from build123d import *

# Parameters (mm, degrees)
SKETCH1_W                = 340
SKETCH1_H                = 400
BOSS_EXTRUDE1_DEPTH      = 20
SKETCH2_W                = 20
SKETCH2_H                = 400
BOSS_EXTRUDE2_DEPTH      = 630
SKETCH3_W                = 300
SKETCH3_H                = 400
BOSS_EXTRUDE3_DEPTH      = 10
BOSS_EXTRUDE4_DEPTH      = 20
BOSS_EXTRUDE4_DEPTH_BACK = 420
SKETCH8_W                = 20
SKETCH8_H                = 780
CUT_EXTRUDE4_DEPTH       = 20
FILLET1_R                = 5
SKETCH10_R               = 3
CUT_EXTRUDE5_DEPTH       = 13
SKETCH11_R               = 3
CUT_EXTRUDE6_DEPTH       = 13
MIRROR5_COPY_1_SKETCH_R  = 3
MIRROR5_COPY_1_DEPTH     = 13


with BuildPart() as part:
    # Sketch1 → Boss-Extrude1 (new body)
    with BuildSketch(Plane(origin=(0, 0, 0), x_dir=(1, 0, 0), z_dir=(0, 1, 0))):
        Rectangle(SKETCH1_W, SKETCH1_H)
    boss_extrude1 = extrude(amount=BOSS_EXTRUDE1_DEPTH)

    # Sketch2 → Boss-Extrude2 (add)
    with BuildSketch(Plane(origin=(0, 20, 0), x_dir=(1, 0, 0), z_dir=(0, 1, 0))):
        with Locations((-160, 0)):
            Rectangle(SKETCH2_W, SKETCH2_H)
    boss_extrude2 = extrude(amount=BOSS_EXTRUDE2_DEPTH)

    # Sketch3 → Boss-Extrude3 (add, symmetric)
    with BuildSketch(Plane(origin=(0, 335, 0), x_dir=(1, 0, 0), z_dir=(0, 1, 0))):
        Rectangle(SKETCH3_W, SKETCH3_H)
    extrude(amount=BOSS_EXTRUDE3_DEPTH, both=True)

    # Mirror1: Boss-Extrude1 across plane
    add(boss_extrude1.mirror(Plane.ZX.offset(335)))

    # Mirror2: Boss-Extrude2 across plane
    add(boss_extrude2.mirror(Plane(origin=(0, 0, 0), x_dir=(0, 0, 1), z_dir=(1, 0, 0))))

    # Sketch8 → Boss-Extrude4 (add, two sides: drawn at the far end of the back side and taken through both)
    with BuildSketch(Plane.XY.offset(200).offset(-BOSS_EXTRUDE4_DEPTH_BACK)):
        with Locations((180, 330)):
            Rectangle(SKETCH8_W, SKETCH8_H)
    extrude(amount=BOSS_EXTRUDE4_DEPTH + BOSS_EXTRUDE4_DEPTH_BACK)

    # Sketch9 → Cut-Extrude4 (cut)
    with BuildSketch(Plane(origin=(190, 0, 0), x_dir=(0, 0, -1), z_dir=(1, 0, 0))):
        with BuildLine():
            Line((-60, 720), (-51.823392624, 695.470177872))
            ThreePointArc((-51.823392624, 695.470177872), (-48.911608517, 691.510062519), (-44.23392624, 690))
            Line((-44.23392624, 690), (44.23392624, 690))
            ThreePointArc((44.23392624, 690), (48.911608517, 691.510062519), (51.823392624, 695.470177872))
            Line((51.823392624, 695.470177872), (60, 720))
            Line((60, 720), (-60, 720))
        make_face()
    extrude(amount=-CUT_EXTRUDE4_DEPTH, mode=Mode.SUBTRACT)

    # Fillet1
    fillet1_edges = [part.edges().sort_by_distance(p)[0] for p in [
        (180, 720, 60),
        (180, 720, -60),
    ]]
    fillet(fillet1_edges, radius=FILLET1_R)

    # Sketch10 → Cut-Extrude5 (cut)
    with BuildSketch(Plane.ZY.offset(170)):
        with Locations((174, 628.5)):
            Circle(SKETCH10_R)
        with Locations((142.5, 628.5)):
            Circle(SKETCH10_R)
        with Locations((111, 628.5)):
            Circle(SKETCH10_R)
    cut_extrude5 = extrude(amount=-CUT_EXTRUDE5_DEPTH, mode=Mode.SUBTRACT)

    # Mirror3: Cut-Extrude5 across plane
    add(cut_extrude5.mirror(Plane.XY), mode=Mode.SUBTRACT)

    # Sketch11 → Cut-Extrude6 (cut)
    with BuildSketch(Plane.XZ):
        with Locations(Location((-124, -140, 0), (0, 0, 270))):
            Circle(SKETCH11_R)
        with Locations(Location((-76, -140, 0), (0, 0, 270))):
            Circle(SKETCH11_R)
    cut_extrude6 = extrude(amount=-CUT_EXTRUDE6_DEPTH, mode=Mode.SUBTRACT)

    # Mirror4: Cut-Extrude6 across plane
    add(cut_extrude6.mirror(Plane(origin=(0, 0, 0), x_dir=(0, 0, 1), z_dir=(1, 0, 0))), mode=Mode.SUBTRACT)

    # Mirror5: Cut-Extrude6 across plane
    add(cut_extrude6.mirror(Plane.XY), mode=Mode.SUBTRACT)

    # Mirror5 copy 1 sketch → Mirror5 copy 1 (cut)
    with BuildSketch(Plane(origin=(0, 0, 0), x_dir=(-1, 0, 0), z_dir=(0, -1, 0))):
        with Locations(Location((-124, -140, 0), (0, 0, 270))):
            Circle(MIRROR5_COPY_1_SKETCH_R)
        with Locations(Location((-76, -140, 0), (0, 0, 270))):
            Circle(MIRROR5_COPY_1_SKETCH_R)
    extrude(amount=-MIRROR5_COPY_1_DEPTH, mode=Mode.SUBTRACT)


solid = part.part
Part model, mm, in its own coordinate system. A direction names the side the tool comes from. Give positions to 0.01 mm unless a question says otherwise; leave off trailing zeros. Order: outer loops, then holes, each group sorted by start corner. A loop starts at its lowest first (then second) coordinate and runs counter-clockwise, first axis right, second up. Notation, with made-up numbers: (51, 80) - (66, 80) arc R19 cw to (66, 110) - close; hole circle Ø1 at (-29.75, 84). An arc over 180 degrees is marked (long way). Use a Markdown table: item, result.
1) Saw through at B-B on x = -41. List the corners of the cut face in (y, z), plus the area to 3 significant figures.
Checked values:
| item | result |
|---|---|
| outline | (0, -200) - (20, -200) - (20, 200) - (0, 200) - close; (325, -200) - (345, -200) - (345, 200) - (325, 200) - close; (650, -200) - (670, -200) - (670, 200) - (650, 200) - close |
| area | 24,000 mm² |
2) Flat gauge pins, fed straight in: P1, Ø7, axis at x = 124, z = -140, coming from the +Y side; P2, Ø1.8, axis at y = 629.5, z = -173.5, coming from the -X side; P3, Ø4, axis at x = -105.5, z = -87.5, coming from the -Y side. Where does each tip first touch, or does it go through?
Checked values:
| item | result |
|---|---|
| P1 | y = 670 |
| P2 | x = -157 |
| P3 | y = 0 |
3) Two-plate mould, pull along Y, no slides. Class faces 1 (the flat face through (180.1, 705.9, -55.3)), 2 (the flat face through (150, 170, 3)), 3 (the flat face through (190, 325, -3)): +Y half, -Y half, draft (parallel to the pull), parting line (faces both ways), or undercut.
Checked values:
| item | result |
|---|---|
| face 1 | +Y half |
| face 2 | undercut |
| face 3 | draft |
4) 3-axis set-ups, long thin cutter, end or side, ignore diameter. For faces 4 (the flat face through (170, 270, 211)), 5 (the flat face through (1, 333, 200)), 6 (the flat face through (1, 333, -200)), 7 (the flat face through (180.1, 706.2, 55.4)), 8 (the flat face through (-150, 495, 3)): which of +Z, -Z, +X, -X, +Y, -Y reach the whole face in a straight line?
Checked values:
| item | result |
|---|---|
| face 4 | -X |
| face 5 | +Z, -X, +Y, -Y |
| face 6 | -Z, -X, +Y, -Y |
| face 7 | +X, -X, +Y |
| face 8 | +Z, -Z |
5) Saw through at C-C on z = -157.5. List the corners of the cut face in (x, y), plus the area to 3 significant figures.
Checked values:
| item | result |
|---|---|
| outline | (-170, 0) - (170, 0) - (170, -60) - (190, -60) - (190, 720) - (170, 720) - (170, 670) - (-170, 670) - close; hole (-150, 20) - (150, 20) - (150, 325) - (-150, 325) - close; hole (-150, 345) - (150, 345) - (150, 650) - (-150, 650) - close |
| area | 60,400 mm² |
6) Saw through at A-A on y = 479. List the corners of the cut face in (x, z), plus the area to 3 significant figures.
Checked values:
| item | result |
|---|---|
| outline | (-170, -200) - (-150, -200) - (-150, 200) - (-170, 200) - close; (150, -200) - (170, -200) - (170, -220) - (190, -220) - (190, 220) - (170, 220) - (170, 200) - (150, 200) - close |
| area | 24,800 mm² |
7) Probe L1, parallel to Y at x = 59.5, z = 140.5; L2, parallel to X at y = 8.75, z = 140; L3, parallel to X at y = 636.5, z = 129. List the from-to ranges inside material, lowest first. Write a range as from..to.
Checked values:
| item | result |
|---|---|
| L1 | 0..20, 325..345, 650..670 |
| L2 | -170..-127, -121..-79, -73..73, 79..121, 127..190 |
| L3 | -170..-150, 150..190 |
